Input: part model. Units: mm. Frame: model coordinates. Face numbers are marked on the shaded views. A direction names the side the tool comes from. Give positions to 0.01 mm unless a question says otherwise; leave off trailing zeros. Loops run counter-clockwise (first coordinate to the right, second up) from the corner with the lowest first, then second, coordinate; pieces in that order, holes last. Notation, with made-up numbers: (81.25, 34.25) -> (140.25, 34.25) arc R8 cw to (140.25, 41.25) -> close; hole circle Ø5 at (77.5, 12). An arc over 180 degrees is marked (long way). Answer as a JSON object with one key per item and string values. Group by question number.
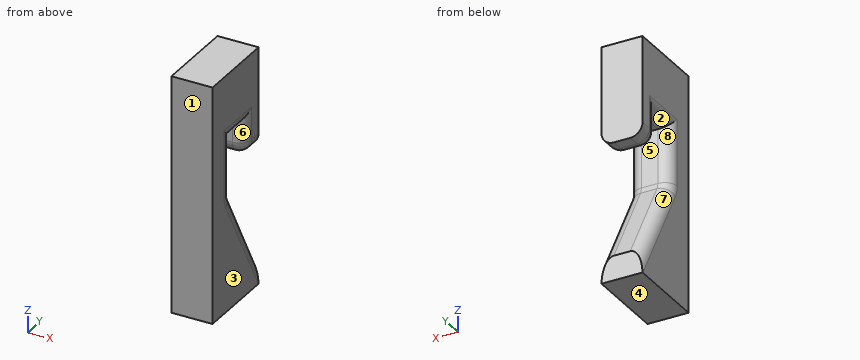
```python
from build123d import *

# Parameters (mm, degrees)
SKETCH2_W           = 10
SKETCH2_H           = 28.8
BOSS_EXTRUDE1_DEPTH = 5
SKETCH3_W           = 3
SKETCH3_H           = 4
CUT_EXTRUDE1_DEPTH  = 31.894012365
FILLET2_R           = 1.5


with BuildPart() as part:
    # Sketch2 → Boss-Extrude1 (new body)
    with BuildSketch(Plane.YZ):
        with Locations((5, 14.4)):
            Rectangle(SKETCH2_W, SKETCH2_H)
    extrude(amount=BOSS_EXTRUDE1_DEPTH)

    # Sketch3 → Cut-Extrude1 (cut, through all)
    with BuildSketch(Plane.YZ.offset(5)):
        with Locations((5.5, 18.8)):
            Rectangle(SKETCH3_W, SKETCH3_H)
        Polygon((7, 16.8), (4, 16.8), (4, 13.8), (10, 3), (10, 16.8), align=None)
    extrude(amount=-CUT_EXTRUDE1_DEPTH, mode=Mode.SUBTRACT)

    # Fillet2
    fillet2_edges = [part.edges().sort_by_distance(p)[0] for p in [
        (5, 4, 17.3),
        (2.5, 4, 13.8),
        (0, 5.5, 20.8),
        (5, 7, 18.8),
        (0, 8.5, 16.8),
        (2.5, 7, 16.8),
        (0, 7, 8.4),
        (0, 4, 17.3),
        (0, 7, 18.8),
        (5, 7, 8.4),
        (5, 8.5, 16.8),
        (5, 5.5, 20.8),
    ]]
    fillet(fillet2_edges, radius=FILLET2_R)


solid = part.part
```
Q1. Pull-direction query (Y, two-part tool) for the marked faces 1, 2 and 3; classes: +Y half, -Y half, draft (parallel to the pull), parting line (faces both ways), or undercut.
Q2. Ray query, probe 1 along Z at (x, y) = (1.4, 7.5); probe 2 along Z at (x, y) = (4.4, 5); probe 3 along X at (y, z) = (2.75, 13.25). Return the intervals inside material, ascending.
Q3. Set-up query: the marked faces 4, 5, 6, 7 and 8. Return all of +Z, -Z, +X, -X, +Y, -Y with unobstructed straight access to the full face (end or side cutting, diameter ignored); none if empty.
Q4. Section A-A on x = 3.15. Return the cut outline in (y, z), then the cut area to 3 significant figures.
Q5. Section B-B on z = 17.5. Return the cut outline in (x, y).
Q6. Section C-C on x = 4.4. Return the cut outline in (y, z).
Q7. Pin query (flat end, axial travel): pin 1 Ø0.6 at (x, y) = (3, 5) entering from -Z. Return the tip coordinate at first contact, or that it passes through.
Numbers:
{
 "1": {"face 1": "-Y half", "face 2": "undercut", "face 3": "draft"},
 "2": {"probe 1": "z = 0 to 7.49, 17.19 to 28.8", "probe 2": "z = 0 to 11.38, 21.1 to 28.8", "probe 3": "x = 0 to 5"},
 "3": {"face 4": "-Z, +X, -X, +Y, -Y", "face 5": "+X, -X", "face 6": "+X", "face 7": "-X, +Y", "face 8": "-X"},
 "4": {"outline": "(0, 0) -> (10, 0) -> (10, 3) -> (4.19, 13.46) arc R1.5 cw to (4, 14.19) -> (4, 20.8) -> (7, 20.8) -> (7, 18.3) arc R1.5 ccw to (8.5, 16.8) -> (10, 16.8) -> (10, 28.8) -> (0, 28.8) -> close", "area": "225 mm²"},
 "5": {"outline": "(0, 0) -> (5, 0) -> (5, 2.5) arc R1.5 ccw to (3.5, 4) -> (1.5, 4) arc R1.5 ccw to (0, 2.5) -> close; (0.23, 8.5) arc R1.27 ccw to (1.5, 7.23) -> (3.5, 7.23) arc R1.27 ccw to (4.77, 8.5) -> (4.77, 10) -> (0.23, 10) -> close"},
 "6": {"outline": "(0, 0) -> (10, 0) -> (10, 2.38) -> (3.93, 13.31) arc R1.8 cw to (3.7, 14.19) -> (3.7, 21.1) -> (7.3, 21.1) -> (7.3, 18.3) arc R1.2 ccw to (8.5, 17.1) -> (10, 17.1) -> (10, 28.8) -> (0, 28.8) -> close"},
 "7": {"pin 1": "stops at z = 0"}
}
